from build123d import *

# Parameters (mm, degrees)
F1_DEPTH = 10


with BuildPart() as f1:
    # F0 (on Top) → F1 (new body)
    with BuildSketch(Plane.XY):
        Polygon((33.02, 26.67), (-33.02, 26.67), (-33.02, -26.67), (33.02, -26.67), (33.02, -24.003), (33.02, 14.147), align=None)
        Polygon((35.56, 11.607), (33.02, 14.147), (33.02, -24.003), (35.56, -21.463), align=None)
    extrude(amount=F1_DEPTH)


solid = f1.part
Geometry: final body of the model. Coordinates: model frame, mm. A direction names the side the tool comes from. Give positions to 0.01 mm unless a question says otherwise; leave off trailing zeros. Write each loop counter-clockwise with the first axis right and the second up, starting at its lowest first coordinate (ties: lowest second). Pieces come first, ordered by that corner, then holes. Notation, with made-up numbers: (71.25, 41) - (128.25, 41) arc R11 cw to (128.25, 45) - close; hole circle Ø4 at (0.5, -25). An arc over 180 degrees is marked (long way). Return JSON: item names as keys, results as strings. Group by question number.
1) Line query: line 1 (X direction, y = 14.5, z = 1); line 2 (X direction, y = 14, z = 5.75). Output: solid intervals per line, ascending.
2) Section A-A on y = 19.5. Return the cut outline in (x, z), plus the area to 3 significant figures.
3) First-contact query: P1, Ø5, axis at y = 20, z = 3, coming from the +X side. Flat tip, straight axial feed; report the tip coordinate or a pass-through.
4) Set-up query: faces 1 (the flat face through (33.02, 20, 5)), 2 (the flat face through (-33.02, 0, 5)), 3 (the flat face through (33.02, -25, 5)). Return all of +Z, -Z, +X, -X, +Y, -Y with unobstructed straight access to the full face (end or side cutting, diameter ignored); none if empty.
Filled in:
{
 "1": {"line 1": "x = -33.02 to 33.02", "line 2": "x = -33.02 to 33.17"},
 "2": {"outline": "(-33.02, 0) - (33.02, 0) - (33.02, 10) - (-33.02, 10) - close", "area": "660 mm^2"},
 "3": {"P1": "stops at x = 33.02"},
 "4": {"face 1": "+Z, -Z, +X, +Y", "face 2": "+Z, -Z, -X, +Y, -Y", "face 3": "+Z, -Z, +X, -Y"}
}
